```python
from build123d import *

# Parameters (mm, degrees)
F1_DEPTH = 120
F3_DEPTH = 5
F4_DEPTH = 5


with BuildPart() as f1:
    # F0 (on Front) → F1 (new body)
    with BuildSketch(Plane.XZ):
        Polygon((0, 80), (0, 0), (5, 0), (5, 70), (9.831525, 85.323638), (61.453404, 159.047322), (57.357644, 161.915204), align=None)
    extrude(amount=F1_DEPTH)

    # F2 (on face) → F3 (join)
    with BuildSketch(Plane(origin=(-37.587705, 0, 26.319194), x_dir=(0, -1, 0), z_dir=(-0.819152, 0, 0.573576))):
        Polygon((0, 65.532164), (0, 165.532164), (-50, 165.532164), align=None)
    extrude(amount=-F3_DEPTH)

    # F2 (on face) → F4 (join)
    with BuildSketch(Plane(origin=(-37.587705, 0, 26.319194), x_dir=(0, -1, 0), z_dir=(-0.819152, 0, 0.573576))):
        Polygon((170, 165.532164), (120, 165.532164), (120, 65.532164), align=None)
    extrude(amount=-F4_DEPTH)


solid = f1.part
```
Design review of the part built by this model. Coordinates are the model's own, in mm. A direction names the side the tool comes from. Give positions to 0.01 mm unless a question says otherwise; leave off trailing zeros. Write each loop counter-clockwise with the first axis right and the second up, starting at its lowest first coordinate (ties: lowest second). Pieces come first, ordered by that corner, then holes.
(1) Wall thickness on line 1 along X through (y, z) = (-44.5, 57); line 2 along X through (y, z) = (-13.5, 72); line 3 along Z through (x, y) = (43, -49): over which ranges is each line inside the solid? List them lowest first.
Checked values:
line 1: x = 0 to 5
line 2: x = 0 to 5.63
line 3: z = 132.69 to 141.41
(2) Tool access review of faces 1 (the face through (5, -59, 35)), 2 (the face through (29.08, -59.16, 121.53)): name each direction out of +Z, -Z, +X, -X, +Y, -Y from which nothing blocks a thin tool from reaching the whole face with its end or side.
Checked values:
face 1: -Z, +X, +Y, -Y
face 2: +Z, -X, +Y, -Y
(3) Add section D-D (z = 49). Give the boundary of the cut face in (x, y), and give its area (3 significant figures).
Checked values:
outline: (0, -120) - (5, -120) - (5, 0) - (0, 0) - close
area: 600 mm2
(4) Add section A-A (y = -66.5). Give the boundary of the cut face in (x, z), and give its area (3 significant figures).
Checked values:
outline: (0, 0) - (5, 0) - (5, 70) - (9.83, 85.32) - (61.45, 159.05) - (57.36, 161.92) - (0, 80) - close
area: 912 mm2
(5) Clearance check with flat-ended pins moving along their axes: pin 1 Ø3 at (x, y) = (27.5, -122.5) entering from +Z; pin 2 Ø12 at (y, z) = (17, 143) entering from +X; pin 3 Ø8 at (y, z) = (-22, 132) entering from +X. State where each tip first meets the part, or that it passes through.
Checked values:
pin 1: stops at z = 121.42
pin 2: stops at x = 54.42
pin 3: stops at x = 45.32
